The figure shows three views and two pictorial views of one solid part (mm, origin at its lowest corner). Answer the questions. A direction names the side the tool comes from. Round coordinates to 2 decimals unless told otherwise and drop trailing zeros.
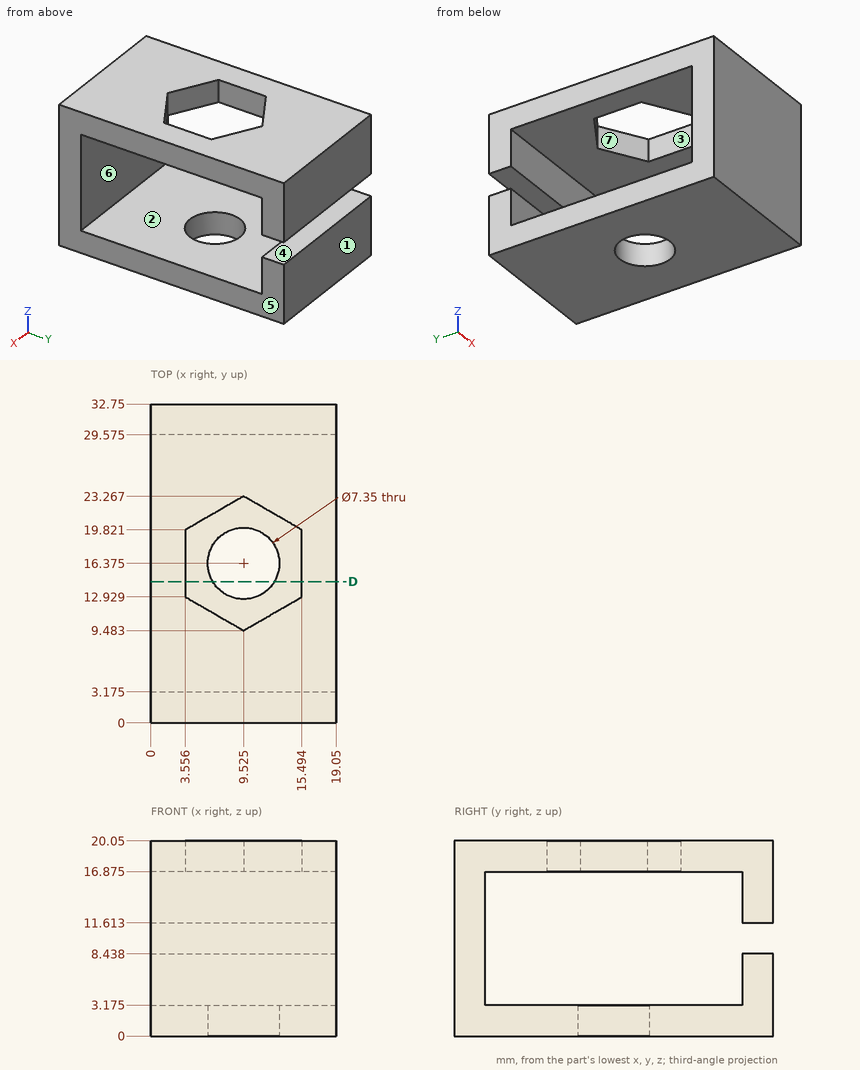
Q1. Flat-ended cylindrical pins translate along their axes: pin 1 Ø8.5 at (x, y) = (9.525, 16.375) entering from +Z (1 decimal); pin 2 Ø2 at (y, z) = (10.5, 5.5) entering from +X. Find the tip coordinate at first contact, or state that the pin passes through.
Verdict:
pin 1: stops at z = 3.2
pin 2: passes through
Q2. Section D-D (y = 14.5) is taken. State how many separate pieces and enclosed holes the cut face has.
Verdict:
separate pieces: 4
enclosed holes: 0
Q3. Determine the mould class of the marked faces 5, 6 and 7 for opening direction X: pulls with the +X half, pulls with the -X half, needs draft (parallel to the pull), parting line crosses it, or undercut.
Verdict:
face 5: pulls with the +X half
face 6: needs draft
face 7: undercut
Q4. Which of the six approach directions +Z, -Z, +X, -X, +Y, -Y give full straight-line access (tool end or side, diameter ignored) to the marked faces 1, 2, 3 and 4?
Verdict:
face 1: +Z, -Z, +X, -X, +Y
face 2: +X, -X
face 3: +Z
face 4: +X, -X, +Y
Q5. Straight lines are drawn through the part: probe 1 along Z at (x, y) = (8.5, 31.5); probe 2 along Y at (x, z) = (11.25, 11) (1 decimal). For each, find the intervals that lie inside material, in ascending order.
Verdict:
probe 1: z = 0 to 8.44, 11.61 to 20.05
probe 2: y = 0 to 3.2
